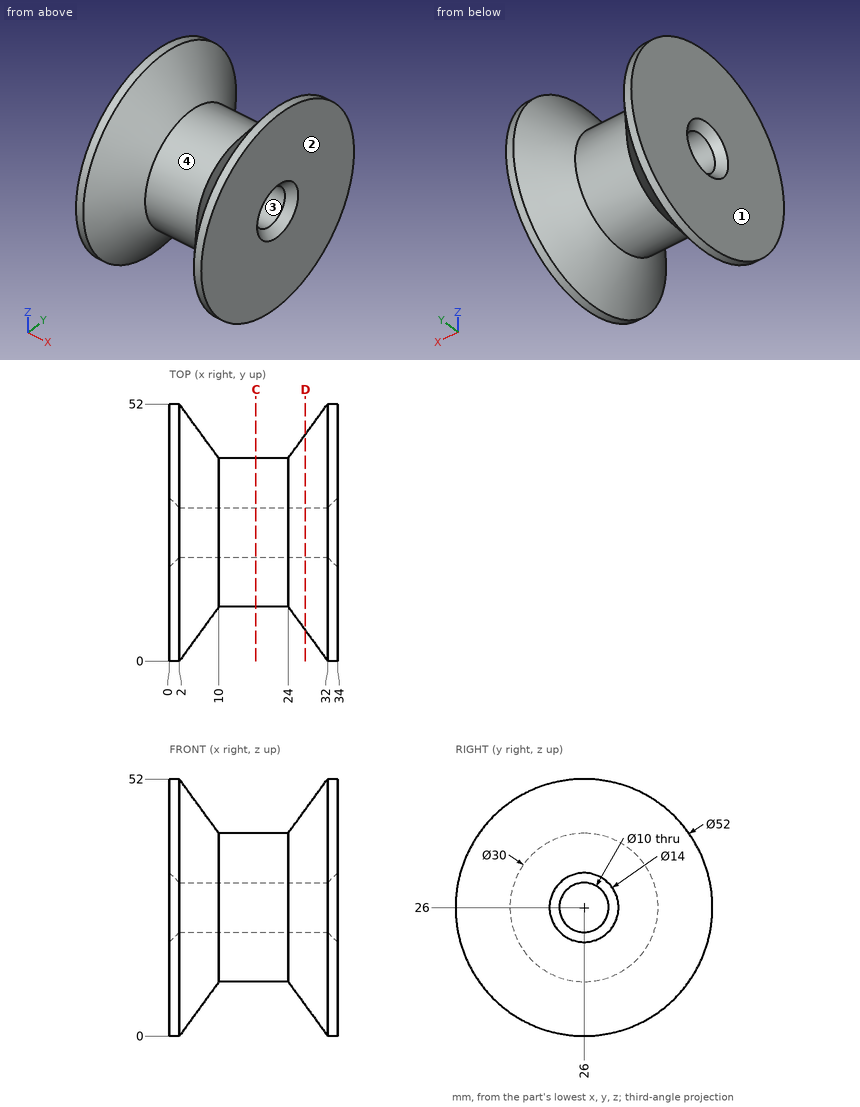
Geometry: see drawing. Coordinates: mm, zero at the bounding-box minimum. Coordinates: 2 decimals unless noted, no trailing zeros. Loops run counter-clockwise (first coordinate to the right, second up) from the corner with the lowest first, then second, coordinate; pieces in that order, holes last. Notation, with made-up numbers: (-34, 58) - (16, 58) arc R18 cw to (16, 63) - close; hole circle Ø3 at (2, 44). An arc over 180 degrees is marked (long way). Return JSON: item names as keys, results as strings.
Q1. Mould query, pull axis X, two halves, no side actions, for the marked faces 1, 2, 3 and 4. Classes: released by +X, released by -X, zero draft, split by the parting line, or undercut.
Results:
{"face 1": "released by -X", "face 2": "released by +X", "face 3": "zero draft", "face 4": "undercut"}
Q2. Section D-D, the plane x = 27.5. Return loops of the section in (y, z) (1 decimal).
Results:
{"outline": "circle Ø39.6 at (26, 26); hole circle Ø10 at (26, 26)"}
Q3. Material intervals for line 1 along Y through (x, z) = (18.25, 26); line 2 along X through (y, z) = (5, 25.5), sorted ascending.
Results:
{"line 1": "11 to 21, 31 to 41", "line 2": "0 to 5.63, 28.37 to 34"}
Q4. Section C-C, the plane x = 17.5. Return loops of the section in (y, z).
Results:
{"outline": "circle Ø30 at (26, 26); hole circle Ø10 at (26, 26)"}
Q5. Contact query for flat-ended pins moving along their axis: P1, Ø4, axis at x = 18.5, z = 33, coming from the -Y side; P2, Ø2, axis at x = 15, y = 35, coming from the +Z side; P3, Ø3, axis at x = 23.5, y = 37, coming from the +Z side; P4, Ø6, axis at y = 26, z = 26, coming from the +X side. Output: stop coordinate, or through.
Results:
{"P1": "y = 11.86", "P2": "z = 38.69", "P3": "z = 38.43", "P4": "through"}
